Input: part model. Units: mm. Frame: model coordinates. Coordinates: 2 decimals unless noted, no trailing zeros. Loops run counter-clockwise (first coordinate to the right, second up) from the corner with the lowest first, then second, coordinate; pieces in that order, holes last. Notation, with made-up numbers: (-14.5, 28) - (40.5, 28) arc R25 ccw to (40.5, 48) - close; hole circle Ø11 at (84, -12.5). An arc over 180 degrees is marked (long way). Use one line per item in the form item = value.
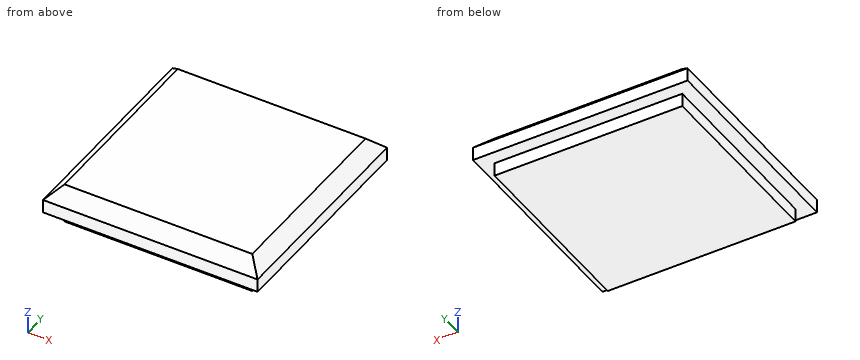
Autodesk Inventor part; units mm, degrees
ref_plane "YZ Plane" through (0, 0, 0) normal (1, 0, 0) x (0, 1, 0)
ref_plane "XZ Plane" through (0, 0, 0) normal (0, 1, 0) x (-1, 0, 0)
ref_plane "XY Plane" through (0, 0, 0) normal (0, 0, 1) x (1, 0, 0)
sketch "Sketch1" plane through (0, 0, 0) normal (0, 0, 1) x (1, 0, 0)
  line L0 (0, 0) -> (50.8, 0)
  line L1 (50.8, 0) -> (50.8, 50.8)
  line L2 (50.8, 50.8) -> (0, 50.8)
  line L3 (0, 50.8) -> (0, 0)
  dimension "d0" = 50.8
  dimension "d1" = 50.8
extrude "Extrusion1" add sketch "Sketch1" along normal blind 3.175
sketch "Sketch2" plane through (0, 0, 0) normal (0, 0, -1) x (-1, 0, 0)
  line L0 (0, 0) -> (-50.8, 0)
  line L1 (-50.8, 0) -> (-50.8, 50.8)
  line L2 (0, 0) -> (-50.8, 0)
  line L3 (-50.8, 0) -> (-50.8, 50.8)
  line L4 (-50.8, 50.8) -> (0, 50.8)
  line L5 (0, 50.8) -> (0, 0)
  line L6 (-3.175, 3.175) -> (-47.625, 3.175)
  line L7 (-47.625, 3.175) -> (-47.625, 47.625)
  line L8 (-47.625, 47.625) -> (-3.175, 47.625)
  line L9 (-3.175, 47.625) -> (-3.175, 3.175)
  dimension "d4" = 3.175
extrude "Extrusion2" add sketch "Sketch2" along normal blind 3.175 contours L6 L7 L8 L9
sketch "Sketch4" plane through (0, 0, 3.175) normal (0, 0, 1) x (1, 0, 0)
  line L0 (0, 0) -> (50.8, 0)
  line L1 (50.8, 0) -> (50.8, 50.8)
  line L2 (0, 0) -> (50.8, 0)
  line L3 (50.8, 0) -> (50.8, 50.8)
  line L4 (50.8, 50.8) -> (0, 50.8)
  line L5 (0, 50.8) -> (0, 0)
extrude "Extrusion4" add sketch "Sketch4" along normal blind 3.175
chamfer "Chamfer1" distance 3.175 angle 45 4 edges at (50.8, 25.4, 6.35) (25.4, 0, 6.35) (0, 25.4, 6.35) (25.4, 50.8, 6.35)
properties part number "End Cap"
Q1. Cut plane D-D, the plane z = -1.5. Return loops of the section in (x, y) (3 decimals).
Check values:
outline = (3.175, 3.175) - (47.625, 3.175) - (47.625, 47.625) - (3.175, 47.625) - close
Q2. Ray query, line 1 along Y through (x, z) = (18, -1.75) (3 decimals); line 2 along Y through (x, z) = (30.5, 5.5) (3 decimals). Return the intervals inside material, ascending. Write a range as [from, to].
Check values:
line_1 = [3.175, 47.625]
line_2 = [2.325, 48.475]
Q3. Cut plane C-C, the plane z = 4.25. Return loops of the section in (x, y) (3 decimals), then the cut area to 3 significant figures.
Check values:
outline = (1.075, 1.075) - (49.725, 1.075) - (49.725, 49.725) - (1.075, 49.725) - close
area = 2,370 mm²
Q4. Cut plane A-A, the plane y = 17.5. Return loops of the section in (x, z) (3 decimals), then the cut area to 3 significant figures.
Check values:
outline = (0, 0) - (3.175, 0) - (3.175, -3.175) - (47.625, -3.175) - (47.625, 0) - (50.8, 0) - (50.8, 3.175) - (47.625, 6.35) - (3.175, 6.35) - (0, 3.175) - close
area = 454 mm²
Q5. First-contact query: P1, Ø1.6, axis at y = 36.5, z = -1.5, coming from the +X side (3 decimals); P2, Ø3.5, axis at x = 33.5, z = -2, coming from the +Y side (3 decimals); P3, Ø1, axis at x = 5, z = -1, coming from the -Y side (3 decimals). Flat tips, straight axial feed; report the tip coordinate or a pass-through.
Check values:
P1 = 47.625
P2 = 47.625
P3 = 3.175
